Here's how the part is built. I have some questions about the finished solid (model axes, mm). A direction names the side the tool comes from. Give positions to 0.01 mm unless a question says otherwise; leave off trailing zeros. Order: outer loops, then holes, each group sorted by start corner. A loop starts at its lowest first (then second) coordinate and runs counter-clockwise, first axis right, second up. Notation, with made-up numbers: M -28.75,67 L 18.25,67 A17 cw 18.25,74 Z; hole C -8.75,-34 d9. An arc over 180 degrees is marked long. One line per item, written item: value. Start each with the question number.
from build123d import *

# Parameters (mm, degrees)
SKETCH1_R           = 1.75
BOSS_EXTRUDE1_DEPTH = 3
BOSS_EXTRUDE2_DEPTH = 3
SKETCH3_R           = 4.5
SKETCH3_R_2         = 3.25
BOSS_EXTRUDE3_DEPTH = 3.2
SKETCH4_R           = 3.25
CUT_EXTRUDE1_DEPTH  = 3
SKETCH6_R           = 7.5
BOSS_EXTRUDE4_DEPTH = 3
SKETCH5_R           = 4.5
CUT_EXTRUDE2_DEPTH  = 7.2
SKETCH7_R           = 7.5
SKETCH7_R_2         = 4.5
BOSS_EXTRUDE5_DEPTH = 2


with BuildPart() as part:
    # Sketch1 → Boss-Extrude1 (new body)
    with BuildSketch(Plane(origin=(0, 0, 0), x_dir=(1, 0, 0), z_dir=(0, 1, 0))):
        with BuildLine():
            Line((0, -4.5), (10, -4.5))
            ThreePointArc((10, -4.5), (14.5, 0), (10, 4.5))
            Line((10, 4.5), (0, 4.5))
            ThreePointArc((0, 4.5), (-4.5, 0), (0, -4.5))
        make_face()
        Circle(SKETCH1_R, mode=Mode.SUBTRACT)
    extrude(amount=BOSS_EXTRUDE1_DEPTH)

    # Sketch2 → Boss-Extrude2 (add)
    with BuildSketch(Plane(origin=(0, 3, 0), x_dir=(1, 0, 0), z_dir=(0, 1, 0))):
        with BuildLine():
            Line((10, 0), (11.688465713, 4.171220869))
            ThreePointArc((11.688465713, 4.171220869), (10.860088975, 4.41704052), (10, 4.5))
            Line((10, 4.5), (6.96685822, 4.5))
            ThreePointArc((6.96685822, 4.5), (8.346615874, -1.181489024), (14.171220869, -1.688465713))
            Line((14.171220869, -1.688465713), (10, 0))
        make_face()
        with BuildLine():
            ThreePointArc((46.064462111, 77.10126181), (43.648814249, 74.646303405), (40.204775529, 74.618506654))
            Line((40.204775529, 74.618506654), (11.688465713, 4.171220869))
            ThreePointArc((11.688465713, 4.171220869), (14.143424118, 1.755573007), (14.171220869, -1.688465713))
            Line((14.171220869, -1.688465713), (46.064462111, 77.10126181))
        make_face()
        with BuildLine():
            ThreePointArc((14.171220869, -1.688465713), (14.143424118, 1.755573007), (11.688465713, 4.171220869))
            Line((11.688465713, 4.171220869), (10, 0))
            Line((10, 0), (14.171220869, -1.688465713))
        make_face()
        with BuildLine():
            Line((11.688465713, 4.171220869), (40.204775529, 74.618506654))
            ThreePointArc((40.204775529, 74.618506654), (37.749817124, 77.034154516), (37.722020373, 80.478193235))
            Line((37.722020373, 80.478193235), (6.96685822, 4.5))
            Line((6.96685822, 4.5), (10, 4.5))
            ThreePointArc((10, 4.5), (10.860088975, 4.41704052), (11.688465713, 4.171220869))
        make_face()
        with BuildLine():
            Line((37.722020373, 80.478193235), (41.893241242, 78.789727523))
            Line((41.893241242, 78.789727523), (46.064462111, 77.10126181))
            ThreePointArc((46.064462111, 77.10126181), (46.310281762, 77.929638548), (46.393241242, 78.789727523))
            ThreePointArc((46.393241242, 78.789727523), (42.753330217, 83.206768043), (37.722020373, 80.478193235))
        make_face()
        with BuildLine():
            Line((46.064462111, 77.10126181), (41.893241242, 78.789727523))
            Line((41.893241242, 78.789727523), (40.204775529, 74.618506654))
            ThreePointArc((40.204775529, 74.618506654), (43.648814249, 74.646303405), (46.064462111, 77.10126181))
        make_face()
        with BuildLine():
            Line((40.204775529, 74.618506654), (41.893241242, 78.789727523))
            Line((41.893241242, 78.789727523), (37.722020373, 80.478193235))
            ThreePointArc((37.722020373, 80.478193235), (37.749817124, 77.034154516), (40.204775529, 74.618506654))
        make_face()
    extrude(amount=-BOSS_EXTRUDE2_DEPTH)

    # Sketch3 → Boss-Extrude3 (add)
    with BuildSketch(Plane(origin=(0, 3, 0), x_dir=(1, 0, 0), z_dir=(0, 1, 0))):
        with Locations((41.893241242, 78.789727523)):
            Circle(SKETCH3_R)
        with Locations((41.893241242, 78.789727523)):
            Circle(SKETCH3_R_2, mode=Mode.SUBTRACT)
    extrude(amount=BOSS_EXTRUDE3_DEPTH)

    # Sketch4 → Cut-Extrude1 (cut)
    with BuildSketch(Plane(origin=(0, 3, 0), x_dir=(1, 0, 0), z_dir=(0, 1, 0))):
        with Locations((41.893241242, 78.789727523)):
            Circle(SKETCH4_R)
    extrude(amount=-CUT_EXTRUDE1_DEPTH, mode=Mode.SUBTRACT)

    # Sketch6 → Boss-Extrude4 (add)
    with BuildSketch(Plane.XZ):
        with Locations((32.137661568, -54.68934028)):
            Circle(SKETCH6_R)
    extrude(amount=-BOSS_EXTRUDE4_DEPTH)

    # Sketch5 → Cut-Extrude2 (cut, through all)
    with BuildSketch(Plane.XZ):
        with Locations((32.137661568, -54.68934028)):
            Circle(SKETCH5_R)
    extrude(amount=-CUT_EXTRUDE2_DEPTH, mode=Mode.SUBTRACT)

    # Sketch7 → Boss-Extrude5 (add)
    with BuildSketch(Plane(origin=(0, 3, 0), x_dir=(1, 0, 0), z_dir=(0, 1, 0))):
        with Locations((32.137661568, 54.68934028)):
            Circle(SKETCH7_R)
        with Locations((32.137661568, 54.68934028)):
            Circle(SKETCH7_R_2, mode=Mode.SUBTRACT)
    extrude(amount=BOSS_EXTRUDE5_DEPTH)


solid = part.part
Item 1: I want a section at C-C on x = 4.5. Write out the boundary of the cut face in (y, z).
Item 2: Will these pins go through, and if not, where does the flat tip stop? P1, Ø4.5, axis at x = 30, z = -53, coming from the +Y side; P2, Ø1, axis at x = 27.5, y = 1.5, coming from the -Z side; P3, Ø4, axis at x = 32.5, z = -39.5, coming from the +Y side; P4, Ø4, axis at x = 41.89, z = -78.79, coming from the +Y side.
Item 3: We'd pull the mould along X, two halves only. Please class faces 4 (the face through (23.975, 1.521, -22.531)), 5 (the face through (41.189, 3.057, -75.617)), 6 (the face through (5, 1, 4.5)): +X half, -X half, draft (parallel to the pull), parting line (faces both ways), or undercut.
Item 4: For faces 1 (the face through (36.542, 2.465, -48.619)), 2 (the face through (-4.5, 1.5, -0.1)), 3 (the face through (4, 1, -4.5)), which set-ups out of +Z, -Z, +X, -X, +Y, -Y let a thin tool reach every point of the face, with its end or its side?
Item 5: I want a section at B-B on y = 2. Write out the boundary of the cut face in (x, z).
Item 6: I want a section at A-A on z = 0. Write out the boundary of the cut face in (x, y).
Item 7: Please list where these lines run through material, in increasing order: probe 1 along Z at (x, y) = (42, 4.5); probe 2 along Z at (x, y) = (3, 1.75); probe 3 along Z at (x, y) = (42, 1.5). Write a range as [from, to].
Answer below:
1. outline: M 0,-4.5 L 3,-4.5 L 3,4.5 L 0,4.5 Z
2. P1: stops at y = 5
2. P2: stops at z = -60.94
2. P3: stops at y = 3
2. P4: passes through
3. face 4: +X half
3. face 5: undercut
3. face 6: draft
4. face 1: +Y
4. face 2: -X, +Y, -Y
4. face 3: -Z, -X, +Y, -Y
5. outline: M 0,-4.5 L 6.97,-4.5 L 25.72,-50.82 A7.5 ccw 30.22,-61.94 L 37.72,-80.48 A4.5 ccw 46.06,-77.1 L 38.56,-58.56 A7.5 ccw 34.06,-47.44 L 14.17,1.69 A4.5 ccw 10,4.5 L 0,4.5 A4.5 ccw Z; hole C 0,0 d3.5; hole C 32.14,-54.69 d9; hole C 41.89,-78.79 d6.5
6. outline: M -4.5,0 L -1.75,0 L -1.75,3 L -4.5,3 Z; M 1.75,0 L 14.85,0 L 14.85,3 L 1.75,3 Z
7. probe 1: z = [-83.29, -82.04], [-75.54, -74.29]
7. probe 2: z = [-4.5, 4.5]
7. probe 3: z = [-83.29, -82.04], [-75.54, -67.06]
